The figure shows three views and two pictorial views of one solid part (mm, origin at its lowest corner). Answer the questions. A direction names the side the tool comes from. Round coordinates to 2 decimals unless told otherwise and drop trailing zeros. Loops run counter-clockwise (first coordinate to the right, second up) from the corner with the lowest first, then second, coordinate; pieces in that order, holes last. Notation, with made-up numbers: (-35, 56) -> (-20, 56) arc R12 ccw to (-20, 79) -> close; hole circle Ø3 at (-21, 35.5). An arc over 180 degrees is marked (long way). Use a Markdown table: item, result. Add a question column.
Q1. Section C-C on y = 11.5 is taken. Give the vertices of the cut face in (x, z), then the cut area to 3 significant figures.
Q2. Consider line 1 (Y direction, x = 16.5, z = 69.5); line 2 (X direction, y = 70, z = 39.5); line 3 (Y direction, x = 25.5, z = 72.5). Determine where each line is inside the solid, lowest interval first.
Q3. Given pin 1 Ø2 at (y, z) = (57.5, 32.5) entering from -X; pin 2 Ø7.5 at (x, z) = (51.5, 36.5) entering from +Y; pin 3 Ø10 at (y, z) = (48, 58) entering from +X, each flat-ended and moving along its own axis, determine where each tip first touches the part or whether it passes through.
Q4. Which of the six approach directions +Z, -Z, +X, -X, +Y, -Y give full straight-line access (tool end or side, diameter ignored) to the marked faces 1, 2 and 3?
Q5. Section A-A on z = 17 is taken. Give the vertices of the cut face in (x, y).
Q6. Section B-B on x = 55.5 is taken. Give the vertices of the cut face in (y, z), then the cut area to 3 significant figures.
Q7. For a pull along Z with two mould halves and no side action, classify the marked faces 4, 5 and 6 as released by +Z, released by -Z, zero draft, split by the parting line, or undercut.
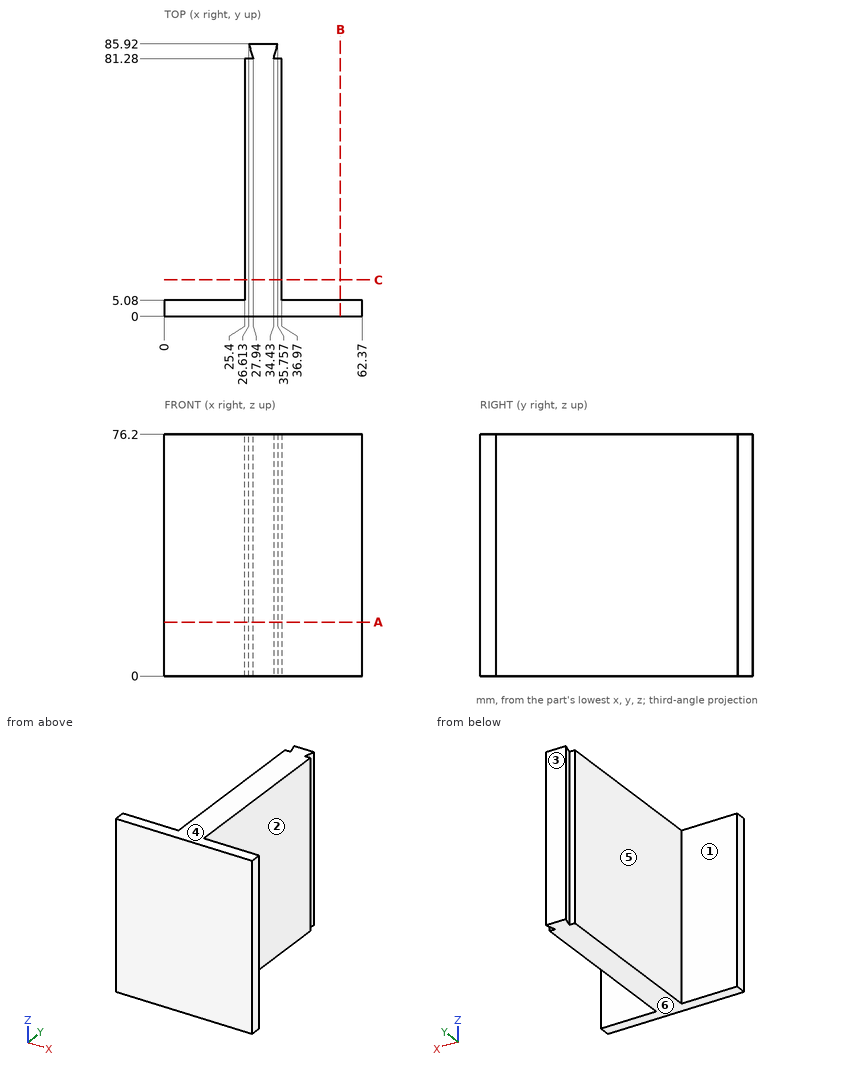
Checked values:
| question | item | result |
|---|---|---|
| 1 | outline | (25.4, 0) -> (36.97, 0) -> (36.97, 76.2) -> (25.4, 76.2) -> close |
| 1 | area | 882 mm2 |
| 2 | line 1 | y = 0 to 5.08 |
| 2 | line 2 | x = 25.4 to 36.97 |
| 2 | line 3 | y = 0 to 81.28 |
| 3 | pin 1 | stops at x = 25.4 |
| 3 | pin 2 | stops at y = 5.08 |
| 3 | pin 3 | stops at x = 36.97 |
| 4 | face 1 | +Z, -Z, -X, +Y |
| 4 | face 2 | +Z, -Z, +X, +Y |
| 4 | face 3 | +Z, -Z, +X, -X, +Y |
| 5 | outline | (0, 0) -> (62.37, 0) -> (62.37, 5.08) -> (36.97, 5.08) -> (36.97, 81.28) -> (34.43, 81.28) -> (35.76, 85.92) -> (26.61, 85.92) -> (27.94, 81.28) -> (25.4, 81.28) -> (25.4, 5.08) -> (0, 5.08) -> close |
| 6 | outline | (0, 0) -> (5.08, 0) -> (5.08, 76.2) -> (0, 76.2) -> close |
| 6 | area | 387 mm2 |
| 7 | face 4 | released by +Z |
| 7 | face 5 | zero draft |
| 7 | face 6 | released by -Z |
